Autodesk Inventor part; units mm, degrees
ref_plane "YZ Plane" through (0, 0, 0) normal (1, 0, 0) x (0, 1, 0)
ref_plane "XZ Plane" through (0, 0, 0) normal (0, 1, 0) x (-1, 0, 0)
ref_plane "XY Plane" through (0, 0, 0) normal (0, 0, 1) x (1, 0, 0)
ref_plane "Work Plane1" through (0, 0, 0) normal (0, 0, 1) x (1, 0, 0)
sketch "Sketch1" plane through (0, 0, 0) normal (0, 0, 1) x (1, 0, 0)
  circle A0 centre (-150, 86.6025) radius 13
  circle A1 centre (0, -173.2051) radius 13
  circle A2 centre (0, -173.2051) radius 11.5
  circle A3 centre (-150, 86.6025) radius 11.5
  circle A4 centre (150, 86.6025) radius 11.5
  circle A5 centre (-150, 86.6025) radius 13
  point P0 (0, 0)
  dimension "d0" = 23
  dimension "d1" = 23
  dimension "d2" = 23
extrude "Extrusion1" add sketch "Sketch1" along normal blind 6 draft -10 contours A3
fillet "Fillet1" radius 2 1 edges at (-160.442, 86.6025, 6)
sketch "Sketch2" plane through (-150, 86.6025, 6) normal (0, 0, 1) x (1, 0, 0)
  circle A0 centre (0, 0) radius 8.7638
  circle A1 centre (0, 0) radius 5
  point P0 (150, -86.6025)
  dimension "d6" = 10
extrude "Extrusion2" cut sketch "Sketch2" against normal blind 3 contours A1
sketch "Sketch3" plane through (-150, 86.6025, 3) normal (0, 0, 1) x (1, 0, 0)
  circle A0 centre (0, 0) radius 5
  circle A1 centre (0, 0) radius 2
  point P0 (150, -86.6025)
  dimension "d9" = 4
extrude "Extrusion3" cut sketch "Sketch3" against normal blind 3 contours A1
sketch "Sketch4" plane through (-150, 86.6025, 6) normal (0, 0, 1) x (1, 0, 0)
  circle A0 centre (0, 0) radius 5
  circle A1 centre (0, 0) radius 8.7638
  circle A2 centre (0, 0) radius 8
  point P0 (150, -86.6025)
  dimension "d12" = 16
extrude "Extrusion4" cut sketch "Sketch4" against normal blind 0.5 contours A2
properties part number "foot" material "Rubber"
Geometry: final body of the model. Coordinates: model frame, mm. A direction names the side the tool comes from. Give positions to 0.01 mm unless a question says otherwise; leave off trailing zeros. Loops run counter-clockwise (first coordinate to the right, second up) from the corner with the lowest first, then second, coordinate; pieces in that order, holes last. Notation, with made-up numbers: (68, 12.25) -> (123, 12.25) arc R20 ccw to (123, 44.25) -> close; hole circle Ø8 at (5.25, 45.5). An arc over 180 degrees is marked (long way). Use one line per item in the form item = value.
Item 1: Section query C-C on z = 5. Output: boundary loops of the cut face in (x, y), and give its area (3 significant figures).
A:
outline = circle Ø20.99 at (-150, 86.6); hole circle Ø10 at (-150, 86.6)
area = 268 mm^2
Item 2: Section query B-B on z = 1.5. Output: boundary loops of the cut face in (x, y).
A:
outline = circle Ø22.47 at (-150, 86.6); hole circle Ø4 at (-150, 86.6)
Item 3: Section query A-A on x = -150. Output: boundary loops of the cut face in (y, z).
A:
outline = (75.1, 0) -> (84.6, 0) -> (84.6, 3) -> (81.6, 3) -> (81.6, 5.5) -> (78.6, 5.5) -> (78.6, 6) -> (77.84, 6) arc R2 ccw to (75.87, 4.35) -> close; (88.6, 0) -> (98.1, 0) -> (97.34, 4.35) arc R2 ccw to (95.37, 6) -> (94.6, 6) -> (94.6, 5.5) -> (91.6, 5.5) -> (91.6, 3) -> (88.6, 3) -> close
Item 4: Draft query along X for faces 3 (the face through (-151.73, 78.79, 5.75)), 4 (the face through (-142, 89, 6)), 5 (the face through (-140.04, 90.73, 4.08)). Return one class per face: pulls with the +X half, pulls with the -X half, needs draft (parallel to the pull), parting line crosses it, or undercut.
A:
face_3 = undercut
face_4 = needs draft
face_5 = parting line crosses it
Item 5: Pin query (flat end, axial travel): P1, Ø5, axis at x = -150.5, y = 90, coming from the +Z side; P2, Ø9, axis at x = -150, y = 86.6, coming from the +Z side; P3, Ø1, axis at x = -151.5, z = 3, coming from the +Y side; P4, Ø3.5, axis at x = -150, y = 86.6, coming from the +Z side. Return the tip coordinate at first contact, or that it passes through.
A:
P1 = 5.5
P2 = 3
P3 = 97.58
P4 = through
Item 6: Access query for faces 1 (the face through (-147.6, 86.8, 0)), 2 (the face through (-154, 83, 5.5)). Directions: +Z, -Z, +X, -X, +Y, -Y. A direction counts if a zero-diameter tool reaches every point of the face in a straight line with its end or side. Return the directions, or none.
A:
face_1 = -Z, +X, -X, +Y, -Y
face_2 = +Z
Item 7: Line query: probe 1 along Z at (x, y) = (-157.5, 88.25); probe 2 along Y at (x, z) = (-150, 1.7); probe 3 along Y at (x, z) = (-150, 4.4). Output: solid intervals per line, ascending.
A:
probe_1 = 0 to 5.5
probe_2 = 75.4 to 84.6, 88.6 to 97.8
probe_3 = 75.88 to 81.6, 91.6 to 97.33
